Check sheet for the drawn part. Datum: minimum x, y, z corner. Units: mm. Give positions to 0.01 mm unless a question says otherwise; leave off trailing zeros. Write each loop counter-clockwise with the first axis right and the second up, starting at its lowest first coordinate (ties: lowest second). Pieces come first, ordered by that corner, then holes. Notation, with made-up numbers: (89.25, 75.25) - (99.25, 75.25) arc R10 cw to (99.25, 84.25) - close; hole circle Ø8 at (32, -3). An arc over 180 degrees is marked (long way). Answer as a JSON object with one key per item and string values. Group by question number.
Item 1: Sectioned sample at A-A, the plane y = 5.25. Record the boundary of the cut face in (x, z) (1 decimal), and give its area (3 significant figures).
Item 2: Sectioned sample at C-C, the plane x = 229. Record the boundary of the cut face in (y, z), and give its area (3 significant figures).
Item 3: Scan lines: line 1 along Z through (x, y) = (157, 4.25) (1 decimal); line 2 along Z through (x, y) = (192.5, 3.75); line 3 along X through (y, z) = (0.5, 100.5) (1 decimal). Record each from-to range of solid material in increasing order. Write a range as [from, to].
Item 4: Go/stop test with flat-tipped pins: pin 1 (5.5 mm diameter, centred on x = 51.06, z = 198.73, fed in from +Y); pin 2 (2 mm diameter, centred on x = 136.5, y = 4.5, fed in from -Z) (1 decimal); pin 3 (1 mm diameter, centred on x = 182, y = 3, fed in from -Z) (1 decimal); pin 4 (2 mm diameter, centred on y = 1.5, z = 22, fed in from +X). Record where each tip stops, or that it passes through.
Item 5: Sectioned sample at B-B, the plane z = 77. Record the boundary of the cut face in (x, y).
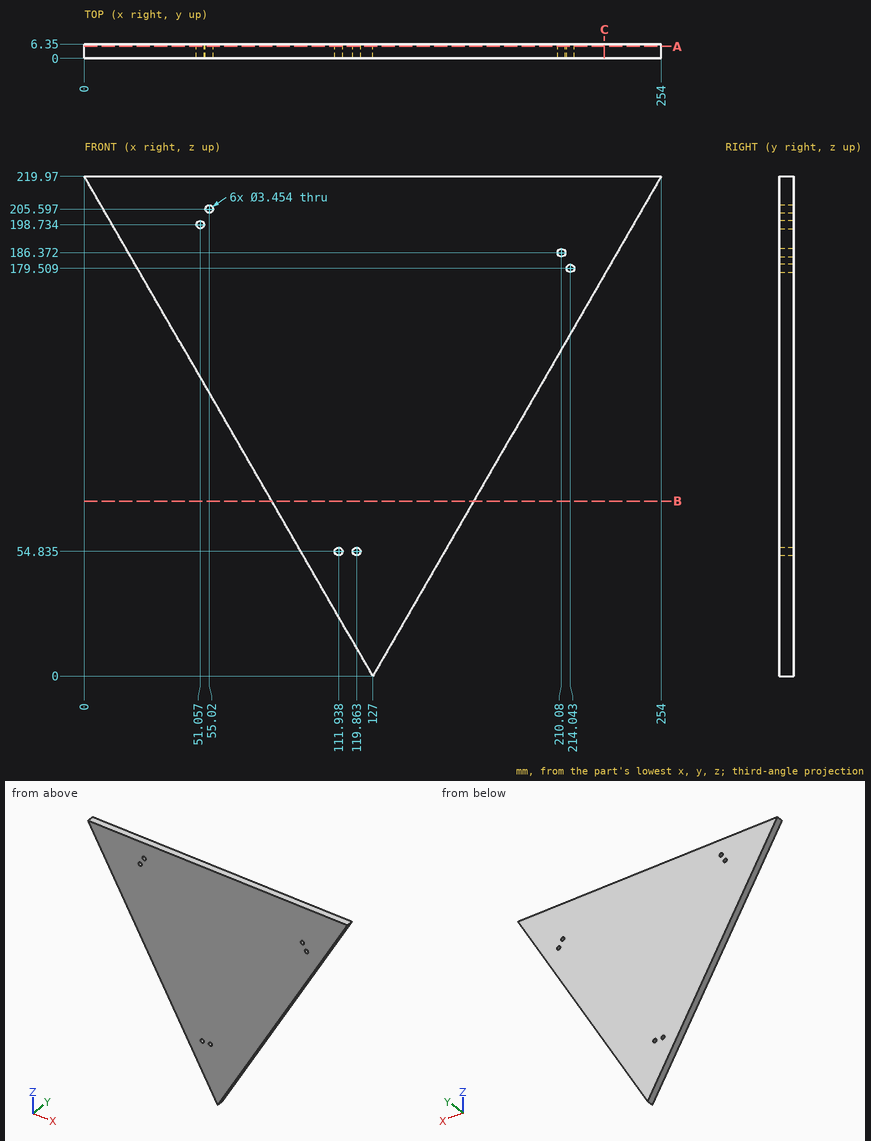
Geometry check:
{
 "1": {"outline": "(0, 220) - (127, 0) - (254, 220) - close; hole circle Ø3.5 at (51.1, 198.7); hole circle Ø3.5 at (55, 205.6); hole circle Ø3.5 at (111.9, 54.8); hole circle Ø3.5 at (119.9, 54.8); hole circle Ø3.5 at (210.1, 186.4); hole circle Ø3.5 at (214, 179.5)", "area": "27,900 mm^2"},
 "2": {"outline": "(0, 176.67) - (6.35, 176.67) - (6.35, 219.97) - (0, 219.97) - close", "area": "275 mm^2"},
 "3": {"line 1": "[52, 220]", "line 2": "[113.45, 219.97]", "line 3": "[69, 185]"},
 "4": {"pin 1": "y = 6.35", "pin 2": "z = 14.7", "pin 3": "z = 94.4", "pin 4": "x = 140.28"},
 "5": {"outline": "(82.54, 0) - (171.46, 0) - (171.46, 6.35) - (82.54, 6.35) - close"}
}
